```python
from build123d import *

# Parameters (mm, degrees)
SKETCH1_R      = 5.125
EXTRUDE1_DEPTH = 10.8


with BuildPart() as part:
    # Sketch1 → Extrude1 (new body)
    with BuildSketch(Plane(origin=(0, 0, 0), x_dir=(1, 0, 0), z_dir=(0, 1, 0))):
        Polygon((10.392304845, 0), (5.196152423, 9), (-5.196152423, 9), (-10.392304845, 0), (-5.196152423, -9), (5.196152423, -9), align=None)
        with Locations(Location((0, 0, 0), (0, 0, 90))):
            Circle(SKETCH1_R, mode=Mode.SUBTRACT)
    extrude(amount=EXTRUDE1_DEPTH)

    # Sketch2 → Cut-Revolve1 (revolve, cut)
    with BuildSketch(Plane.XY, mode=Mode.PRIVATE) as cut_revolve1_sk:
        Polygon((-8.3, 10.8), (-10.392304845, 9.592007234), (-10.392304845, 10.8), align=None)
        Polygon((-10.392304845, 1.207992766), (-8.3, 0), (-10.392304845, 0), align=None)
    revolve(cut_revolve1_sk.sketch.rotate(Axis((0, 0, 0), (0, 1, 0)), 270), axis=Axis((0, 0, 0), (0, 1, 0)), mode=Mode.SUBTRACT)


solid = part.part
```
Input: part model. Units: mm. Frame: model coordinates. Coordinates: 2 decimals unless noted, no trailing zeros. Write each loop counter-clockwise with the first axis right and the second up, starting at its lowest first coordinate (ties: lowest second). Pieces come first, ordered by that corner, then holes. Notation, with made-up numbers: (53.25, 48) - (81.25, 48) arc R28 cw to (81.25, 84) - close; hole circle Ø1 at (-6, 67.5). An arc over 180 degrees is marked (long way). Put each result on its own line as item: value. Start each with the question number.
1) Contact query for a flat-ended pin moving along its axis: pin 1 (4 mm diameter, centred on x = 1.5, z = 1, fed in from -Y). Output: stop coordinate, or through.
2) Cut plane A-A (x = 0). Return the cut outline in (y, z) (3 decimals).
3) Ray query, L1, parallel to X at y = 8, z = -2.5; L2, parallel to Z at x = 1.5, y = 1; L3, parallel to Z at x = 2.5, y = 8. Return the intervals inside material, ascending.
4) Cut plane B-B (y = 9). Return the cut outline in (x, z) (3 decimals).
Resolved:
1. pin 1: passes through
2. outline: (0, -8.3) - (0.404, -9) - (10.396, -9) - (10.8, -8.3) - (10.8, -5.125) - (0, -5.125) - close; (0, 5.125) - (10.8, 5.125) - (10.8, 8.3) - (10.396, 9) - (0.404, 9) - (0, 8.3) - close
3. L1: x = -8.95 to -4.47, 4.47 to 8.95
3. L2: z = -9 to -4.9, 4.9 to 9
3. L3: z = -9 to -4.47, 4.47 to 9
4. outline: (-10.392, 0) - (-5.196, -9) - (5.196, -9) - (10.392, 0) - (5.196, 9) - (-5.196, 9) - close; hole circle Ø10.25 at (0, 0)
